from build123d import *

# Parameters (mm, degrees)
SKETCH_1_R                    = 64
SKETCH_1_R_2                  = 49
EXTRUDE_1_DEPTH               = 52
SKETCH_13_R                   = 49
SKETCH_13_R_2                 = 35.5
EXTRUDE_3_DEPTH               = 11.2
HOLE_WIZARD_M4_11_D           = 4.3
HOLE_WIZARD_M4_11_CBORE_D     = 8
HOLE_WIZARD_M4_11_CBORE_DEPTH = 4.6
SKETCH_18_R                   = 74
SKETCH_18_R_2                 = 56
EXTRUDE_4_DEPTH               = 13
SKETCH_25_R                   = 4
EXTRUDE_7_DEPTH               = 5
SKETCH_28_R                   = 4
EXTRUDE_8_DEPTH               = 5
CUT_EXTRUDE_2_DEPTH           = 81
FILLET_4_R                    = 10
FILLET_5_R                    = 10
RIB_1_REACH                   = 128.89
SKETCH_32_WALL_W              = 297.523252796
SKETCH_32_WALL_H              = 10
RIB_2_REACH                   = 128.89
SKETCH_33_WALL_W              = 297.523252796
SKETCH_33_WALL_H              = 10
RIB_7_REACH                   = 128.89
SKETCH_34_WALL_W              = 297.523252796
SKETCH_34_WALL_H              = 10
RIB_9_REACH                   = 128.89
SKETCH_35_WALL_W              = 297.523252796
SKETCH_35_WALL_H              = 10
SKETCH_36_R                   = 56
SKETCH_36_R_2                 = 55
EXTRUDE_9_DEPTH               = 13
SKETCH_37_R                   = 55.5
CUT_EXTRUDE_3_DEPTH           = 8.5


with BuildPart() as part:
    # 草图1 → 凸台-拉伸1 (new body)
    with BuildSketch(Plane(origin=(0, 0, 0), x_dir=(1, 0, 0), z_dir=(0, 1, 0))):
        with Locations(Location((0, 0, 0), (0, 0, 90))):
            Circle(SKETCH_1_R)
        with Locations(Location((0, 0, 0), (0, 0, 90))):
            Circle(SKETCH_1_R_2, mode=Mode.SUBTRACT)
    extrude(amount=EXTRUDE_1_DEPTH)

    # 草图13 → 凸台-拉伸3 (add)
    with BuildSketch(Plane.XZ):
        with Locations(Location((0, 0, 0), (0, 0, 270))):
            Circle(SKETCH_13_R)
        with Locations(Location((0, 0, 0), (0, 0, 270))):
            Circle(SKETCH_13_R_2, mode=Mode.SUBTRACT)
    extrude(amount=-EXTRUDE_3_DEPTH)

    # M4 六角圆柱头螺钉的柱形沉头孔11 (through all)
    with Locations(Plane.XZ):
        with Locations((-38.980021964, -22.484614467), (38.970883682, -22.50044944), (-38.970883682, 22.50044944), (38.978008551, 22.483453082)):
            CounterBoreHole(HOLE_WIZARD_M4_11_D / 2, HOLE_WIZARD_M4_11_CBORE_D / 2, HOLE_WIZARD_M4_11_CBORE_DEPTH)

    # 草图18 → 凸台-拉伸4 (add)
    with BuildSketch(Plane(origin=(0, 52, 0), x_dir=(1, 0, 0), z_dir=(0, 1, 0))):
        with Locations(Location((0, 0, 0), (0, 0, 90))):
            Circle(SKETCH_18_R)
        with Locations(Location((0, 0, 0), (0, 0, 90))):
            Circle(SKETCH_18_R_2, mode=Mode.SUBTRACT)
    extrude(amount=EXTRUDE_4_DEPTH)

    # 草图25 → 凸台-拉伸7 (add)
    with BuildSketch(Plane.XZ):
        with BuildLine():
            Line((-74, 57.021028333), (-74, 70))
            ThreePointArc((-74, 70), (-71.071067812, 77.071067812), (-64, 80))
            Line((-64, 80), (64, 80))
            ThreePointArc((64, 80), (71.071067812, 77.071067812), (74, 70))
            Line((74, 70), (74, 57.021028333))
            ThreePointArc((74, 57.021028333), (72.870108332, 52.403542201), (69.735764364, 48.82950789))
            Line((69.735764364, 48.82950789), (52.425730834, 36.708891926))
            ThreePointArc((52.425730834, 36.708891926), (0, 64), (-52.425730834, 36.708891926))
            Line((-52.425730834, 36.708891926), (-69.735764364, 48.82950789))
            ThreePointArc((-69.735764364, 48.82950789), (-72.870108332, 52.403542201), (-74, 57.021028333))
        make_face()
        with Locations(Location((-64, 70, 0), (0, 0, 270))):
            Circle(SKETCH_25_R, mode=Mode.SUBTRACT)
        with Locations(Location((64, 70, 0), (0, 0, 270))):
            Circle(SKETCH_25_R, mode=Mode.SUBTRACT)
    extrude(amount=-EXTRUDE_7_DEPTH)

    # 草图28 → 凸台-拉伸8 (add)
    with BuildSketch(Plane.XZ):
        with BuildLine():
            Line((-52.425730834, -36.708891926), (-69.735764364, -48.82950789))
            ThreePointArc((-69.735764364, -48.82950789), (-72.870108332, -52.403542201), (-74, -57.021028333))
            Line((-74, -57.021028333), (-74, -70))
            ThreePointArc((-74, -70), (-71.071067812, -77.071067812), (-64, -80))
            Line((-64, -80), (64, -80))
            ThreePointArc((64, -80), (71.071067812, -77.071067812), (74, -70))
            Line((74, -70), (74, -57.021028333))
            ThreePointArc((74, -57.021028333), (72.870108332, -52.403542201), (69.735764364, -48.82950789))
            Line((69.735764364, -48.82950789), (52.425730834, -36.708891926))
            ThreePointArc((52.425730834, -36.708891926), (0, -64), (-52.425730834, -36.708891926))
        make_face()
        with Locations(Location((-64, -70, 0), (0, 0, 270))):
            Circle(SKETCH_28_R, mode=Mode.SUBTRACT)
        with Locations(Location((64, -70, 0), (0, 0, 270))):
            Circle(SKETCH_28_R, mode=Mode.SUBTRACT)
    extrude(amount=-EXTRUDE_8_DEPTH)

    # 草图14 → 切除-拉伸2 (cut)
    with BuildSketch(Plane.XY):
        Polygon((0, 0), (20, 0), (20, 16.2), (-20, 16.2), (-20, 0), align=None)
    extrude(amount=CUT_EXTRUDE_2_DEPTH, mode=Mode.SUBTRACT)

    # 圆角4
    fillet_4_edges = [part.edges().sort_by_distance(p)[0] for p in [
        (-20, 2.5, 80),
    ]]
    fillet(fillet_4_edges, radius=FILLET_4_R)

    # 圆角5
    fillet_5_edges = [part.edges().sort_by_distance(p)[0] for p in [
        (20, 2.5, 80),
    ]]
    fillet(fillet_5_edges, radius=FILLET_5_R)

    # 草图32 wall → 筋1 (add, up to next)
    with BuildSketch(Plane(origin=(61.080747599, 23, 42.769199908), x_dir=(-0.414672953097, 0.86240308464, -0.290357127642), z_dir=(0.706439249784, 0.506222203783, 0.494654087986)), mode=Mode.PRIVATE) as rib_1_sk1:
        with Locations((0, 5)):
            Rectangle(SKETCH_32_WALL_W, SKETCH_32_WALL_H)
    rib_1_tool1 = extrude(rib_1_sk1.sketch, amount=-RIB_1_REACH, mode=Mode.PRIVATE) - part.part
    add(rib_1_tool1.solids().sort_by_distance((61.080747599, 23, 42.769199908))[0])

    # 草图33 wall → 筋2 (add, up to next)
    with BuildSketch(Plane(origin=(-61.080747599, 23, 42.769199908), x_dir=(-0.414672953097, -0.86240308464, 0.290357127642), z_dir=(-0.706439249784, 0.506222203783, 0.494654087986)), mode=Mode.PRIVATE) as rib_2_sk1:
        with Locations((0, 5)):
            Rectangle(SKETCH_33_WALL_W, SKETCH_33_WALL_H)
    rib_2_tool1 = extrude(rib_2_sk1.sketch, amount=-RIB_2_REACH, mode=Mode.PRIVATE) - part.part
    add(rib_2_tool1.solids().sort_by_distance((-61.080747599, 23, 42.769199908))[0])

    # 草图34 wall → 筋7 (add, up to next)
    with BuildSketch(Plane(origin=(-61.080747599, 23, -42.769199908), x_dir=(0.414672953097, 0.86240308464, 0.290357127642), z_dir=(-0.706439249784, 0.506222203783, -0.494654087986)), mode=Mode.PRIVATE) as rib_7_sk1:
        with Locations((0, 5)):
            Rectangle(SKETCH_34_WALL_W, SKETCH_34_WALL_H)
    rib_7_tool1 = extrude(rib_7_sk1.sketch, amount=-RIB_7_REACH, mode=Mode.PRIVATE) - part.part
    add(rib_7_tool1.solids().sort_by_distance((-61.080747599, 23, -42.769199908))[0])

    # 草图35 wall → 筋9 (add, up to next)
    with BuildSketch(Plane(origin=(61.080747599, 23, -42.769199908), x_dir=(0.414672953097, -0.86240308464, -0.290357127642), z_dir=(0.706439249784, 0.506222203783, -0.494654087986)), mode=Mode.PRIVATE) as rib_9_sk1:
        with Locations((0, 5)):
            Rectangle(SKETCH_35_WALL_W, SKETCH_35_WALL_H)
    rib_9_tool1 = extrude(rib_9_sk1.sketch, amount=-RIB_9_REACH, mode=Mode.PRIVATE) - part.part
    add(rib_9_tool1.solids().sort_by_distance((61.080747599, 23, -42.769199908))[0])

    # 草图36 → 凸台-拉伸9 (add)
    with BuildSketch(Plane(origin=(0, 52, 0), x_dir=(1, 0, 0), z_dir=(0, 1, 0))):
        Circle(SKETCH_36_R)
        with Locations(Location((0, 0, 0), (0, 0, 270))):
            Circle(SKETCH_36_R_2, mode=Mode.SUBTRACT)
    extrude(amount=EXTRUDE_9_DEPTH)

    # 草图37 → 切除-拉伸3 (cut)
    with BuildSketch(Plane(origin=(0, 65, 0), x_dir=(1, 0, 0), z_dir=(0, 1, 0))):
        with Locations(Location((0, 0, 0), (0, 0, 270))):
            Circle(SKETCH_37_R)
    extrude(amount=-CUT_EXTRUDE_3_DEPTH, mode=Mode.SUBTRACT)


solid = part.part
Here's how the part is built. I have some questions about the finished solid (model axes, mm). A direction names the side the tool comes from. Coordinates: 2 decimals unless noted, no trailing zeros. Write each loop counter-clockwise with the first axis right and the second up, starting at its lowest first coordinate (ties: lowest second). Pieces come first, ordered by that corner, then holes.
1) If we section it at D-D (x = 24): List the corners of the cut face in (y, z) for me, plus the area to 3 significant figures.
Filled in:
outline: (0, -80) - (5, -80) - (5, -59.33) - (52, -59.33) - (52, -70) - (65, -70) - (65, -50.04) - (56.5, -50.04) - (56.5, -49.49) - (52, -49.49) - (52, -42.72) - (11.2, -42.72) - (11.2, -26.16) - (0, -26.16) - close; (0, 26.16) - (11.2, 26.16) - (11.2, 42.72) - (52, 42.72) - (52, 49.49) - (56.5, 49.49) - (56.5, 50.04) - (65, 50.04) - (65, 70) - (52, 70) - (52, 59.33) - (5, 59.33) - (5, 78) - (0, 78) - close
area: 2,820 mm2
2) Thinking about a two-plate mould opening in Z: for faces 4 (the face through (53.277, 17.191, -49.512)), 5 (the face through (46.798, 60.81, 29.836)), 6 (the face through (52.044, 15.605, 48.649)), 7 (the face through (-40.96, 7.95, 21.68)), which applies, +Z half, -Z half, draft (parallel to the pull), parting line (faces both ways), or undercut?
Filled in:
face 4: -Z half
face 5: undercut
face 6: +Z half
face 7: undercut
3) Which directions (+Z, -Z, +X, -X, +Y, -Y) give clear straight access to the entire face, cutting with the end or side of a thin tool? Please do faces 1 (the face through (-41.92, 2.27, 25.2)), 2 (the face through (24.51, 25.64, -59.12)), 3 (the face through (72.9, 2.46, -52.46)).
Filled in:
face 1: -Y
face 2: none
face 3: +X, +Y, -Y
4) I'm going to push flat-ended pins straight in: pin 1 (5 mm diameter, centred on x = 38.98, z = 22.48, fed in from +Y); pin 2 (5 mm diameter, centred on x = 38.98, z = 22.48, fed in from -Y); pin 3 (8 mm diameter, centred on x = 10.5, y = 34, fed in from +Z). Where does each tip first touch, or does it pass through?
Filled in:
pin 1: stops at y = 11.2
pin 2: stops at y = 4.6
pin 3: stops at z = 63.67
5) If we section it at C-C (y = 28.5): List the corners of the cut face in (x, z) for me, plus the area to 3 significant figures.
Filled in:
outline: (-58.44, -40.92) - (-52.7, -49.11) - (-46.05, -44.45) arc R64 ccw to (46.05, -44.45) - (52.7, -49.11) - (58.44, -40.92) - (52.43, -36.71) arc R64 ccw to (52.43, 36.71) - (58.44, 40.92) - (52.7, 49.11) - (46.05, 44.45) arc R64 ccw to (-46.05, 44.45) - (-52.7, 49.11) - (-58.44, 40.92) - (-52.43, 36.71) arc R64 ccw to (-52.43, -36.71) - close; hole circle Ø98 at (0, 0)
area: 5,630 mm2
6) If we section it at A-A (x = 0): List the corners of the cut face in (y, z) for me.
Filled in:
outline: (0, -80) - (5, -80) - (5, -64) - (52, -64) - (52, -74) - (65, -74) - (65, -55.5) - (56.5, -55.5) - (56.5, -55) - (52, -55) - (52, -49) - (11.2, -49) - (11.2, -35.5) - (0, -35.5) - close; (16.2, 49) - (52, 49) - (52, 55) - (56.5, 55) - (56.5, 55.5) - (65, 55.5) - (65, 74) - (52, 74) - (52, 64) - (16.2, 64) - close
7) If we section it at B-B (z = -31): List the corners of the cut face in (x, y) for me.
Filled in:
outline: (-67.19, 52) - (-55.99, 52) - (-55.99, 0) - (-17.3, 0) - (-17.3, 11.2) - (-37.95, 11.2) - (-37.95, 52) - (-45.43, 52) - (-45.43, 56.5) - (-46.04, 56.5) - (-46.04, 65) - (-67.19, 65) - close; (17.3, 0) - (55.99, 0) - (55.99, 52) - (67.19, 52) - (67.19, 65) - (46.04, 65) - (46.04, 56.5) - (45.43, 56.5) - (45.43, 52) - (37.95, 52) - (37.95, 11.2) - (17.3, 11.2) - close
8) If I drill on line 1 (X direction, y = 1.65, z = 70); line 2 (X direction, y = 59, z = 1.5); line 3 (Z direction, x = 56, y = 8.5), over which ranges is the centre line in solid material (lowest first)?
Filled in:
line 1: x = -74 to -68, -60 to -20, 20 to 60, 68 to 74
line 2: x = -73.98 to -55.48, 55.48 to 73.98
line 3: z = -51.42 to -39.21, -30.98 to 30.98, 39.21 to 51.42
